Check sheet for the modelled part. Datum: model origin and axes. Units: mm. Give positions to 0.01 mm unless a question says otherwise; leave off trailing zeros. Write each loop counter-clockwise with the first axis right and the second up, starting at its lowest first coordinate (ties: lowest second). Pieces come first, ordered by that corner, then holes. Notation, with made-up numbers: (-40, 27) -> (2, 27) arc R31 ccw to (2, 63) -> close; hole circle Ø5 at (56.25, 85.5). An arc over 180 degrees is marked (long way). Use a Markdown table: item, result. Add a question column.
1. Cross-section at A-A (x = 228.6). Enter the section's corners in (y, z).
2. Cross-section at B-B (z = -342.9). Enter the section's corners in (x, y), then the cut area to 3 significant figures.
3. Gauge pin test, flat end, axial feed: P1, Ø5, axis at x = 198.5, z = -340, coming from the -Y side. Record the tip position at first contact, or that the pin passes through.
4. Cross-section at C-C (y = -3.65). Enter the section's corners in (x, z).
5. Scan lines: probe 1 along X at (y, z) = (-2.35, -342.9); probe 2 along Z at (x, y) = (-44.45, -2.3); probe 3 along Z at (x, y) = (-67.5, -1.25). Record each from-to range of solid material in increasing order. Write a range as [from, to].
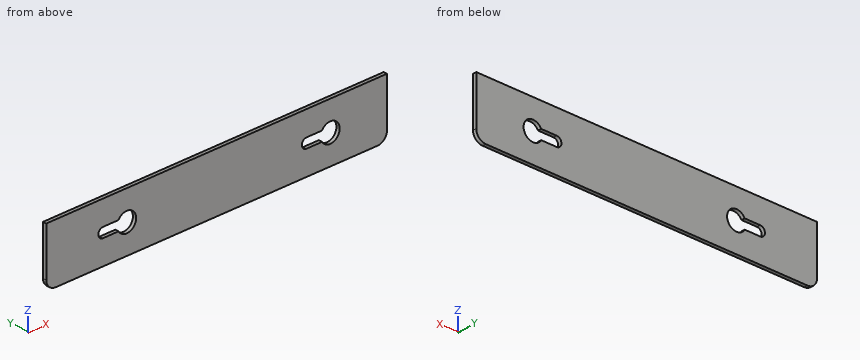
from build123d import *

# Parameters (mm, degrees)
F1_DEPTH = 4.7498


# Not quite as in the source:
# - a feature names something its author has since deleted; it is built from what else it names


with BuildPart() as f1:
    # F0 (on Front) → F1 (new body)
    with BuildSketch(Plane.XZ):
        with BuildLine():
            Line((304.8, -368.3), (304.8, -304.8))
            Line((304.8, -304.8), (0, -304.8))
            Line((0, -304.8), (-152.4, -304.8))
            Line((-152.4, -304.8), (-152.4, -368.3))
            ThreePointArc((-152.4, -368.3), (-148.6802561211, -377.2802561211), (-139.7, -381))
            Line((-139.7, -381), (292.1, -381))
            ThreePointArc((292.1, -381), (301.0802561211, -377.2802561211), (304.8, -368.3))
        make_face()
        with BuildLine():
            ThreePointArc((-55.4485226281, -336.55), (-31.75, -342.9), (-55.4485226281, -349.25))
            Line((-55.4485226281, -349.25), (-76.2, -349.25))
            ThreePointArc((-76.2, -349.25), (-82.55, -342.9), (-76.2, -336.55))
            Line((-76.2, -336.55), (-55.4485226281, -336.55))
        make_face(mode=Mode.SUBTRACT)
        with BuildLine():
            ThreePointArc((217.6014773719, -336.55), (241.3, -342.9), (217.6014773719, -349.25))
            Line((217.6014773719, -349.25), (196.85, -349.25))
            ThreePointArc((196.85, -349.25), (190.5, -342.9), (196.85, -336.55))
            Line((196.85, -336.55), (217.6014773719, -336.55))
        make_face(mode=Mode.SUBTRACT)
    extrude(amount=F1_DEPTH)


solid = f1.part
Worked answers:
| question | item | result |
|---|---|---|
| 1 | outline | (-4.75, -381) -> (0, -381) -> (0, -355.6) -> (-4.75, -355.6) -> close; (-4.75, -330.2) -> (0, -330.2) -> (0, -304.8) -> (-4.75, -304.8) -> close |
| 2 | outline | (-152.4, -4.75) -> (-82.55, -4.75) -> (-82.55, 0) -> (-152.4, 0) -> close; (-31.75, -4.75) -> (190.5, -4.75) -> (190.5, 0) -> (-31.75, 0) -> close; (241.3, -4.75) -> (304.8, -4.75) -> (304.8, 0) -> (241.3, 0) -> close |
| 2 | area | 1,690 mm² |
| 3 | P1 | passes through |
| 4 | outline | (-152.4, -368.3) arc R12.7 ccw to (-139.7, -381) -> (292.1, -381) arc R12.7 ccw to (304.8, -368.3) -> (304.8, -304.8) -> (-152.4, -304.8) -> close; hole (-76.2, -349.25) -> (-55.45, -349.25) arc R12.7 ccw (long way) to (-55.45, -336.55) -> (-76.2, -336.55) arc R6.35 ccw to start; hole (196.85, -349.25) -> (217.6, -349.25) arc R12.7 ccw (long way) to (217.6, -336.55) -> (196.85, -336.55) arc R6.35 ccw to start |
| 5 | probe 1 | x = [-152.4, -82.55], [-31.75, 190.5], [241.3, 304.8] |
| 5 | probe 2 | z = [-381, -355.6], [-330.2, -304.8] |
| 5 | probe 3 | z = [-381, -349.25], [-336.55, -304.8] |
